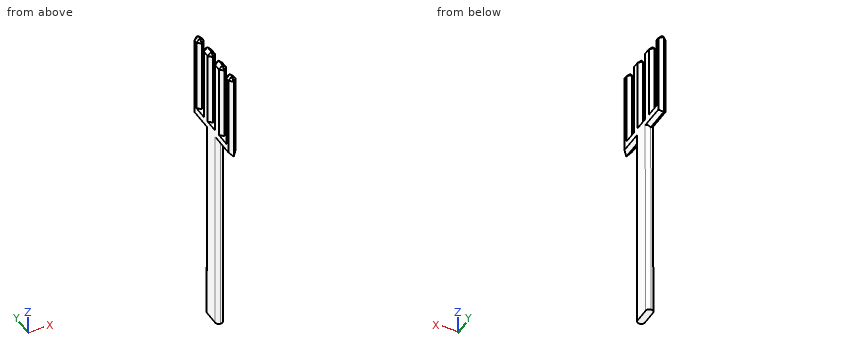
```python
from build123d import *

# Parameters (mm, degrees)
F1_DEPTH = 2.54
F2_R     = 1.26999
F3_SIZE  = 1.26999


# Not quite as in the source:
# - a fillet or chamfer is up to 0.001 mm smaller than in the source, because OpenCascade refuses the exact size


with BuildPart() as f1:
    # F0 (on Right) → F1 (new body)
    with BuildSketch(Plane.YZ):
        Polygon((41.3628902497, -55.5398087384), (48.9828902497, -55.5398087384), (49.3619268672, -55.5398087384), (48.9828902497, 16.8501912616), (57.8728902497, 16.8501912616), (57.8728902497, 20.5470483008), (57.8728902497, 47.7535999747), (54.0628902497, 47.7535999747), (54.0628902497, 20.5470483008), (51.5228902497, 20.5470483008), (51.5228902497, 47.7535999747), (46.4428902497, 47.7535999747), (46.4428902497, 20.5470483008), (43.9028902497, 20.5470483008), (43.9028902497, 47.7535999747), (38.8228902497, 47.7535999747), (38.8228902497, 20.5470483008), (36.2828902497, 20.5470483008), (36.2828902497, 47.7535999747), (32.4728902497, 47.7535999747), (32.4728902497, 16.8502441253), (41.3628902497, 16.8502441253), align=None)
    extrude(amount=F1_DEPTH)

    # F2 (radius 1.27 in the source; OpenCascade refuses exactly that, so slightly less here)
    f2_edges = [f1.edges().sort_by_distance(p)[0] for p in [
        (0, 49.172409, -19.344809),
        (2.54, 41.36289, -19.344782),
        (0, 41.36289, -19.344782),
        (2.54, 49.172409, -19.344809),
    ]]
    fillet(f2_edges, radius=F2_R)

    # F3 (size 1.27 in the source; OpenCascade refuses exactly that, so slightly less here)
    f3_edges = [f1.edges().sort_by_distance(p)[0] for p in [
        (0, 53.42789, 16.850191),
        (2.54, 53.42789, 16.850191),
        (0, 36.91789, 16.850244),
        (2.54, 36.91789, 16.850244),
        (0, 57.87289, 32.301896),
        (2.54, 57.87289, 32.301896),
        (2.54, 54.06289, 34.150324),
        (0, 54.06289, 34.150324),
        (2.54, 36.28289, 34.150324),
        (0, 36.28289, 34.150324),
        (2.54, 43.90289, 34.150324),
        (0, 43.90289, 34.150324),
        (2.54, 51.52289, 34.150324),
        (0, 51.52289, 34.150324),
        (2.54, 32.47289, 32.301922),
        (0, 32.47289, 32.301922),
        (2.54, 38.82289, 34.150324),
        (0, 38.82289, 34.150324),
        (2.54, 46.44289, 34.150324),
        (0, 46.44289, 34.150324),
        (1.27, 51.52289, 47.7536),
        (1.27, 46.44289, 47.7536),
        (0, 48.98289, 47.7536),
        (2.54, 48.98289, 47.7536),
        (1.27, 43.90289, 47.7536),
        (1.27, 38.82289, 47.7536),
        (0, 41.36289, 47.7536),
        (2.54, 41.36289, 47.7536),
        (1.27, 36.28289, 47.7536),
        (1.27, 32.47289, 47.7536),
        (0, 34.37789, 47.7536),
        (2.54, 34.37789, 47.7536),
        (1.27, 57.87289, 47.7536),
        (1.27, 54.06289, 47.7536),
        (0, 55.96789, 47.7536),
        (2.54, 55.96789, 47.7536),
    ]]
    chamfer(f3_edges, length=F3_SIZE)


solid = f1.part
```
Here's how the part is built. I have some questions about the finished solid (model axes, mm). Give positions to 0.01 mm unless a question says otherwise; leave off trailing zeros. Order: outer loops, then holes, each group sorted by start corner. A loop starts at its lowest first (then second) coordinate and runs counter-clockwise, first axis right, second up. Notation, with made-up numbers: (-7.5, -15.5) - (15.5, -15.5) arc R17 ccw to (15.5, 14.5) - close; hole circle Ø11 at (13.5, 27.25). An arc over 180 degrees is marked (long way). Answer as a JSON object with one key per item and string values. Group by question number.
Item 1: For P1, Ø0.8, axis at x = 1, y = 45.5, coming from the +Z side; P2, Ø1, axis at x = 0.5, y = 40, coming from the -Z side; P3, Ø1.5, axis at x = 1.5, z = -31.5, coming from the +Y side, each with a flat end and sliding along its axis, tell me the tip position at first contact or that it passes through.
Item 2: Please list where these lines run through material, in increasing order: probe 1 along Y at (x, z) = (2.05, 25); probe 2 along Y at (x, z) = (2, 35); probe 3 along Z at (x, y) = (0.25, 45.5).
Item 3: If we section it at A-A on z = 39: Give the number of separate pieces and of enclosed holes in the cut face, and give its area (3 significant figures).
Item 4: If we section it at B-B on x = 2: Please give me the cut outline in (y, z).
Result set:
{
 "1": {"P1": "z = 20.55", "P2": "z = 17.12", "P3": "y = 49.24"},
 "2": {"probe 1": "33.25 to 35.5, 39.6 to 43.12, 47.22 to 50.74, 54.84 to 57.09", "probe 2": "33.2 to 35.55, 39.55 to 43.17, 47.17 to 50.79, 54.79 to 57.14", "probe 3": "-55.54 to 20.55"},
 "3": {"separate pieces": "4", "enclosed holes": "0", "area": "32.3 mm²"},
 "4": {"outline": "(33.2, 17.58) - (41.59, 17.58) - (41.59, -55.54) - (49.13, -55.54) - (48.75, 17.58) - (57.14, 17.58) - (57.14, 46.48) - (56.6, 47.02) - (55.33, 47.02) - (54.79, 46.48) - (54.79, 20.55) - (50.79, 20.55) - (50.79, 46.48) - (50.25, 47.02) - (47.71, 47.02) - (47.17, 46.48) - (47.17, 20.55) - (43.17, 20.55) - (43.17, 46.48) - (42.63, 47.02) - (40.09, 47.02) - (39.55, 46.48) - (39.55, 20.55) - (35.55, 20.55) - (35.55, 46.48) - (35.01, 47.02) - (33.74, 47.02) - (33.2, 46.48) - close"}
}
